Here's how the part is built. I have some questions about the finished solid (model axes, mm). A direction names the side the tool comes from. Give positions to 0.01 mm unless a question says otherwise; leave off trailing zeros. Write each loop counter-clockwise with the first axis right and the second up, starting at its lowest first coordinate (ties: lowest second). Pieces come first, ordered by that corner, then holes. Notation, with made-up numbers: M 8.25,15 L 37.25,15 A32 ccw 37.25,53 Z; hole C -13,75 d6. An arc over 180 degrees is marked long. Answer as CSV lines item,"result". Start each with the question number.
Q1. If I drill on line 1 along X through (y, z) = (10.5, -14); line 2 along Y through (x, z) = (24.5, -26); line 3 along Y through (x, z) = (16.5, -30), over which ranges is the centre line in solid material (lowest first)?
Q2. Suppose I cut it at C-C (y = -4). Write out the boundary of the cut face in (x, z).
Q3. Suppose I cut it at A-A (y = 15). Write out the boundary of the cut face in (x, z), then the cut area to 3 significant figures.
Q4. Suppose I cut it at D-D (z = -24). Write out the boundary of the cut face in (x, y), then the cut area to 3 significant figures.
Q5. Suppose I cut it at B-B (x = 12.5). Write out the boundary of the cut face in (y, z).
Q6. On a 3-axis mill with a long thin cutter (end or side, diameter ignored), from which of +Z, -Z, +X, -X, +Y, -Y can I reach the whole of each face in a straight line? I mean faces 4 (the cylindrical face through (24.65, -2.67, 17.67)), 5 (the flat face through (15, 11.627, -8)), 6 (the flat face through (30, 6.627, -9)), 7 (the cylindrical face through (9, 17.76, 28.61)). Say none if no direction works.
Q7. Thinking about a two-plate mould opening in X: for faces 1 (the flat face through (25, 11.627, 29)), 2 (the flat face through (25, -18.373, -11)), 3 (the cylindrical face through (47.148, -13.303, -33.309)), which applies, +X half, -X half, draft (parallel to the pull), parting line (faces both ways), or undercut?
Q8. For pin 1 (3 mm diameter, centred on x = 20, z = 12, fed in from +Y); pin 2 (4 mm diameter, centred on y = -7, z = 24, fed in from -X); pin 3 (1 mm diameter, centred on x = 12, z = -20.5, fed in from +Y); pin 4 (3 mm diameter, centred on x = 39, z = 21.5, fed in from -Y), each with a flat end and sliding along its axis, tell me the tip position at first contact or that it passes through.
```python
from build123d import *

# Parameters (mm, degrees)
SALIENTE_EXTRUIR1_DEPTH = 50
CORTAR_EXTRUIR1_DEPTH   = 85.263005614
REDONDEO1_R             = 10
REDONDEO2_R             = 10
REDONDEO3_R             = 10
REDONDEO4_R             = 10
CROQUIS5_R              = 15
SALIENTE_EXTRUIR5_DEPTH = 20
CROQUIS7_R              = 10
CORTAR_EXTRUIR3_DEPTH   = 5
CROQUIS9_R              = 5
CORTAR_EXTRUIR4_DEPTH   = 15


with BuildPart() as part:
    # Croquis1 → Saliente-Extruir1 (new body)
    with BuildSketch(Plane(origin=(0, 0, 0), x_dir=(0, 0, -1), z_dir=(1, 0, 0))):
        with BuildLine():
            Line((-33.684210526, 31.626794258), (-33.684210526, 1.626794258))
            ThreePointArc((-33.684210526, 1.626794258), (-27.82634615, -12.515341365), (-13.684210526, -18.373205742))
            Line((-13.684210526, -18.373205742), (36.315789474, -18.373205742))
            Line((36.315789474, -18.373205742), (36.315789474, -8.373205742))
            Line((36.315789474, -8.373205742), (-3.684210526, -8.373205742))
            ThreePointArc((-3.684210526, -8.373205742), (-17.82634615, -2.515341365), (-23.684210526, 11.626794258))
            Line((-23.684210526, 11.626794258), (-23.684210526, 31.626794258))
            Line((-23.684210526, 31.626794258), (-33.684210526, 31.626794258))
        make_face()
    extrude(amount=SALIENTE_EXTRUIR1_DEPTH)

    # Croquis2 → Cortar-Extruir1 (cut, through all)
    with BuildSketch(Plane(origin=(0, 0, 23.684210526), x_dir=(-1, 0, 0), z_dir=(0, 0, -1))):
        with BuildLine():
            Line((-35, 23.626794258), (-15, 23.626794258))
            ThreePointArc((-15, 23.626794258), (-9, 17.626794258), (-15, 11.626794258))
            Line((-15, 11.626794258), (-35, 11.626794258))
            ThreePointArc((-35, 11.626794258), (-41, 17.626794258), (-35, 23.626794258))
        make_face()
    extrude(amount=-CORTAR_EXTRUIR1_DEPTH, mode=Mode.SUBTRACT)

    # Redondeo1
    redondeo1_edges = [part.edges().sort_by_distance(p)[0] for p in [
        (50, 31.626794258, 28.684210526),
    ]]
    fillet(redondeo1_edges, radius=REDONDEO1_R)

    # Redondeo2
    redondeo2_edges = [part.edges().sort_by_distance(p)[0] for p in [
        (0, 31.626794258, 28.684210526),
    ]]
    fillet(redondeo2_edges, radius=REDONDEO2_R)

    # Redondeo3
    redondeo3_edges = [part.edges().sort_by_distance(p)[0] for p in [
        (50, -13.373205742, -36.315789474),
    ]]
    fillet(redondeo3_edges, radius=REDONDEO3_R)

    # Redondeo4
    redondeo4_edges = [part.edges().sort_by_distance(p)[0] for p in [
        (0, -13.373205742, -36.315789474),
    ]]
    fillet(redondeo4_edges, radius=REDONDEO4_R)

    # Croquis5 → Saliente-Extruir5 (add)
    with BuildSketch(Plane(origin=(0, -8.373205742, 0), x_dir=(1, 0, 0), z_dir=(0, 1, 0))):
        with Locations(Location((25, 11.315789474, 0), (0, 0, 270))):
            Circle(CROQUIS5_R)
    extrude(amount=SALIENTE_EXTRUIR5_DEPTH)

    # Croquis7 → Cortar-Extruir3 (cut)
    with BuildSketch(Plane(origin=(0, 11.626794258, 0), x_dir=(1, 0, 0), z_dir=(0, 1, 0))):
        with Locations(Location((25, 11.315789474, 0), (0, 0, 270))):
            Circle(CROQUIS7_R)
    extrude(amount=-CORTAR_EXTRUIR3_DEPTH, mode=Mode.SUBTRACT)

    # Croquis9 → Cortar-Extruir4 (cut)
    with BuildSketch(Plane(origin=(0, 6.626794258, 0), x_dir=(1, 0, 0), z_dir=(0, 1, 0))):
        with Locations(Location((25, 11.315789474, 0), (0, 0, 270))):
            Circle(CROQUIS9_R)
    extrude(amount=-CORTAR_EXTRUIR4_DEPTH, mode=Mode.SUBTRACT)


solid = part.part
```
Resolved:
1,line 1,"10.24 to 15.37, 34.63 to 39.76"
1,line 2,"-18.37 to 11.63"
1,line 3,"-18.37 to -8.37"
2,outline,"M 0,16.17 L 50,16.17 L 50,32.88 L 0,32.88 Z; C 25,-11.32 d30; hole C 25,-11.32 d10"
3,outline,"M 0,23.68 L 9.61,23.68 L 9.61,33.68 L 0,33.68 Z; M 40.39,23.68 L 50,23.68 L 50,33.68 L 40.39,33.68 Z"
3,area,"192 mm^2"
4,outline,"M 0,-18.37 L 50,-18.37 L 50,-8.37 L 33.01,-8.37 L 33.01,11.63 L 16.99,11.63 L 16.99,-8.37 L 0,-8.37 Z"
4,area,"820 mm^2"
5,outline,"M -18.37,-36.32 L -8.37,-36.32 L -8.37,-19.61 L 11.63,-19.61 L 11.63,-3.02 L -8.37,-3.02 L -8.37,3.68 A20 cw 11.63,23.68 L 12.17,23.68 L 12.17,33.68 L 1.63,33.68 A20 ccw -18.37,13.68 Z; M 23.08,23.68 L 31.63,23.68 L 31.63,33.68 L 23.08,33.68 Z"
6,face 4,"+X, -X, +Y"
6,face 5,"-Z, +X, -X, +Y"
6,face 6,"+Y"
6,face 7,"+Z, -Z"
7,face 1,"undercut"
7,face 2,"draft"
7,face 3,"+X half"
8,pin 1,"y = -5.8"
8,pin 2,"x = 0"
8,pin 3,"y = -8.37"
8,pin 4,"y = -17.35"
